Check sheet for the modelled part. Datum: model origin and axes. Units: mm. Face numbers are marked on the shaded views. A direction names the side the tool comes from. Give positions to 0.01 mm unless a question says otherwise; leave off trailing zeros. Order: outer loops, then holes, each group sorted by start corner. A loop starts at its lowest first (then second) coordinate and runs counter-clockwise, first axis right, second up.
Item 1: Access from +Z, -Z, +X, -X, +Y, -Y to the whole of each face (thin tool, end or side, straight path). Record for the marked faces 1, 2 and 3.
Item 2: Sectioned sample at B-B on y = 15.5. Record the boundary of the cut face in (x, z), and give its area (3 significant figures).
Item 3: Sectioned sample at A-A on x = 12. Record the boundary of the cut face in (y, z).
Item 4: Release check for a two-part mould opening along X. For the marked faces 4, 5 and 6 record: released by +X, released by -X, zero draft, split by the parting line, or undercut.
Item 5: Sectioned sample at C-C on z = 3. Count the separate pieces of the cut face and the enclosed holes in it, and give its area (3 significant figures).
Item 6: Material ranges on line 1 along X through (y, z) = (54, 7); line 2 along Z through (x, y) = (6.5, 79); line 3 along Y through (x, z) = (15.5, 5), recorded low to high.
Item 7: Gauge pin test, flat ends, axial feed: P1, Ø3.5, axis at x = 12.5, z = 3, coming from the -Y side; P2, Ø4, axis at x = 14.5, y = 11.5, coming from the -Z side; P3, Ø4, axis at y = 55, z = 3.5, coming from the +X side; P4, Ø2.5, axis at y = 15, z = 4.5, coming from the -X side. Record the tip position at first contact, or that the pin passes through.
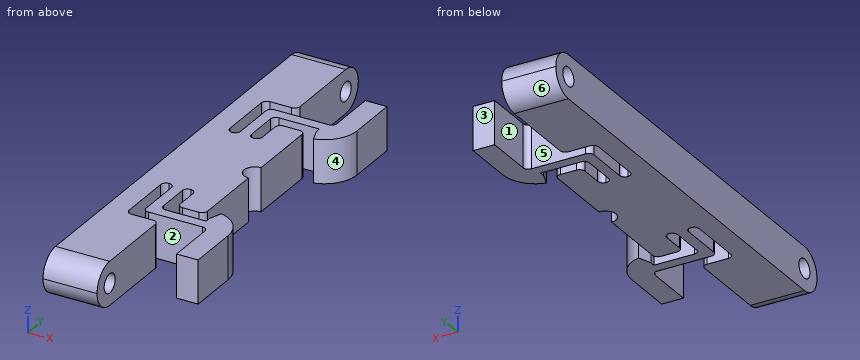
from build123d import *

# Parameters (mm, degrees)
F0_W        = 4
F0_H        = 8
F0_H_2      = 2
F0_W_2      = 5.5
F0_H_3      = 3.5
F1_DEPTH    = 8
F2_R        = 3.99999
F3_T1_DEPTH = 37.8956518578
F4_T1_DEPTH = 21.1532650868
F5_T1_DEPTH = 21.1532650868
F7_DEPTH    = 8
F8_R        = 0.99999
F9_R        = 1.75
F10_DEPTH   = 10


# Not quite as in the source:
# - a fillet or chamfer that OpenCascade refuses, or shapes differently, is made with other operations: its cross-section is extruded or revolved along the edge and cut away or added
# - a fillet or chamfer is up to 0.001 mm smaller than in the source, because OpenCascade refuses the exact size


with BuildPart() as f1:
    # F0 (on Top) → F1 (new body)
    with BuildSketch(Plane.XY):
        Polygon((0, 83), (0, 0), (10, 0), (10, 10), (10, 19.5), (8, 19.5), (4, 19.5), (4, 31.5), (6, 31.5), (8, 31.5), (10, 31.5), (10, 25.5), (15, 25.5), (15, 57.5), (10, 57.5), (10, 51.5), (8, 51.5), (6, 51.5), (4, 51.5), (4, 63.5), (8, 63.5), (10, 63.5), (10, 73), (10, 83), align=None)
        with Locations((20, 67.5)):
            Rectangle(F0_W, F0_H)
        with Locations((20, 62.5)):
            Rectangle(F0_W, F0_H_2)
        with Locations((19.25, 57.75)):
            Rectangle(F0_W_2, F0_H_3)
        with Locations((19.25, 25.25)):
            Rectangle(F0_W_2, F0_H_3)
        with Locations((20, 20.5)):
            Rectangle(F0_W, F0_H_2)
        with Locations((20, 15.5)):
            Rectangle(F0_W, F0_H)
        Polygon((8, 23.5), (8, 21.5), (18, 21.5), (22, 21.5), (22, 23.5), (16.5, 23.5), (15, 23.5), align=None)
        Polygon((6, 21.5), (8, 21.5), (8, 23.5), (8, 25.5), (8, 31.5), (6, 31.5), align=None)
        Polygon((8, 59.5), (8, 61.5), (6, 61.5), (6, 51.5), (8, 51.5), (8, 57.5), align=None)
        Polygon((18, 61.5), (8, 61.5), (8, 59.5), (15, 59.5), (16.5, 59.5), (22, 59.5), (22, 61.5), align=None)
    extrude(amount=F1_DEPTH)

    # F2 (radius 4 in the source; OpenCascade refuses exactly that, so slightly less here)
    f2_edges = [f1.edges().sort_by_distance(p)[0] for p in [
        (5, 83, 8),
        (5, 0, 8),
        (5, 0, 0),
        (5, 83, 0),
    ]]
    fillet(f2_edges, radius=F2_R)

    # F3: fillet of radius 6 on 2 edges, made by hand

    # F3_s2 → F3_t1 (cut)
    with BuildSketch(Plane.XY.offset(-14.9478259289)):
        with BuildLine():
            ThreePointArc((22, 61.9791303716), (20.4158804332, 57.9171111692), (16.5, 56))
            Line((16.5, 56), (22, 56))
            Line((22, 56), (22, 61.9791303716))
        make_face()
        with BuildLine():
            ThreePointArc((22, 21.0208696284), (20.4158804332, 25.0828888308), (16.5, 27))
            Line((16.5, 27), (22, 27))
            Line((22, 27), (22, 21.0208696284))
        make_face()
    extrude(amount=F3_T1_DEPTH, mode=Mode.SUBTRACT)

    # F4: chamfer of 0.5 x 2.5 on 1 edges, made by hand

    # F4_s2 → F4_t1 (cut)
    with BuildSketch(Plane.XY.offset(-6.5766325434)):
        with BuildLine():
            Line((17.379363756, 56.0377654524), (16.466798813, 58.6304434947))
            Line((16.466798813, 58.6304434947), (16.416798813, 58.6304434947))
            ThreePointArc((16.416798813, 58.6304434947), (16.45, 57.3152217474), (16.45, 56))
            Line((16.45, 56), (16.5041666667, 55.9501739136))
            ThreePointArc((16.5041666667, 55.9501739136), (16.9421943049, 56.0029468158), (17.3905817774, 55.9890401407))
            Line((17.3905817774, 55.9890401407), (17.379363756, 56.0377654524))
        make_face()
    extrude(amount=F4_T1_DEPTH, mode=Mode.SUBTRACT)

    # F5: chamfer of 0.5 x 2.5 on 1 edges, made by hand

    # F5_s2 → F5_t1 (cut)
    with BuildSketch(Plane.XY.offset(-6.5766325434)):
        with BuildLine():
            Line((16.466798813, 24.3695565053), (17.379363756, 26.9622345476))
            Line((17.379363756, 26.9622345476), (17.3905817774, 27.0109598593))
            ThreePointArc((17.3905817774, 27.0109598593), (16.9421943049, 26.9970531842), (16.5041666667, 27.0498260864))
            Line((16.5041666667, 27.0498260864), (16.45, 27))
            ThreePointArc((16.45, 27), (16.45, 25.6847782526), (16.416798813, 24.3695565053))
            Line((16.416798813, 24.3695565053), (16.466798813, 24.3695565053))
        make_face()
    extrude(amount=F5_T1_DEPTH, mode=Mode.SUBTRACT)

    # F6 (on face) → F7 (cut)
    with BuildSketch(Plane(origin=(0, 0, 0), x_dir=(1, 0, 0), z_dir=(0, 0, -1))):
        with BuildLine():
            Line((15, -43.5), (15, -39.5))
            ThreePointArc((15, -39.5), (13, -41.5), (15, -43.5))
        make_face()
    extrude(amount=-F7_DEPTH, mode=Mode.SUBTRACT)

    # F8 (radius 1 in the source; OpenCascade refuses exactly that, so slightly less here)
    f8_edges = [f1.edges().sort_by_distance(p)[0] for p in [
        (18, 21.5, 4),
        (6, 21.5, 4),
        (4, 19.5, 4),
        (10, 19.5, 4),
        (8, 23.5, 4),
        (15, 25.5, 4),
        (10, 25.5, 4),
        (8, 31.5, 4),
        (10, 31.5, 4),
        (6, 31.5, 4),
        (4, 31.5, 4),
        (6, 51.5, 4),
        (10, 51.5, 4),
        (18, 61.5, 4),
        (6, 61.5, 4),
        (10, 57.5, 4),
        (15, 57.5, 4),
        (8, 59.5, 4),
        (4, 51.5, 4),
        (8, 51.5, 4),
        (4, 63.5, 4),
        (10, 63.5, 4),
    ]]
    fillet(f8_edges, radius=F8_R)

    # F9 (on face) → F10 (cut)
    with BuildSketch(Plane(origin=(0, 0, 0), x_dir=(0, -1, 0), z_dir=(-1, 0, 0))):
        with Locations((-79, 4)):
            Circle(F9_R)
        with Locations((-4, 4)):
            Circle(F9_R)
    extrude(amount=-F10_DEPTH, mode=Mode.SUBTRACT)


solid = f1.part
Report:
1. face 1: +Z, -Z, +Y
1. face 2: +Z, -Z
1. face 3: +Z, -Z, +X, +Y
2. outline: (0, 0) - (10, 0) - (10, 8) - (0, 8) - close; (18, 0) - (22, 0) - (22, 8) - (18, 8) - close
2. area: 112 mm2
3. outline: (21.5, 0) - (23.5, 0) - (23.5, 8) - (21.5, 8) - close; (25.5, 0) - (57.5, 0) - (57.5, 8) - (25.5, 8) - close; (59.5, 0) - (61.5, 0) - (61.5, 8) - (59.5, 8) - close
4. face 4: released by +X
4. face 5: undercut
4. face 6: zero draft
5. separate pieces: 3
5. enclosed holes: 0
5. area: 978 mm2
6. line 1: x = 0 to 4, 6 to 8, 10 to 15
6. line 2: z = 0 to 2.25, 5.75 to 8
6. line 3: y = 21.5 to 23.5, 59.5 to 61.5
7. P1: stops at y = 21.5
7. P2: passes through
7. P3: stops at x = 19.35
7. P4: stops at x = 0
